Verification items for this drawing (mm, ordinates from the low corner). Give positions to 0.01 mm unless a question says otherwise; leave off trailing zeros. Loops run counter-clockwise (first coordinate to the right, second up) from the corner with the lowest first, then second, coordinate; pieces in that order, holes last. Notation, with made-up numbers: M -6,-16.5 L 0,-16.5 A30 ccw 0,20.5 Z; hole C 10.25,35 d10. An arc over 180 degrees is marked long. Use a Markdown table: item, result.
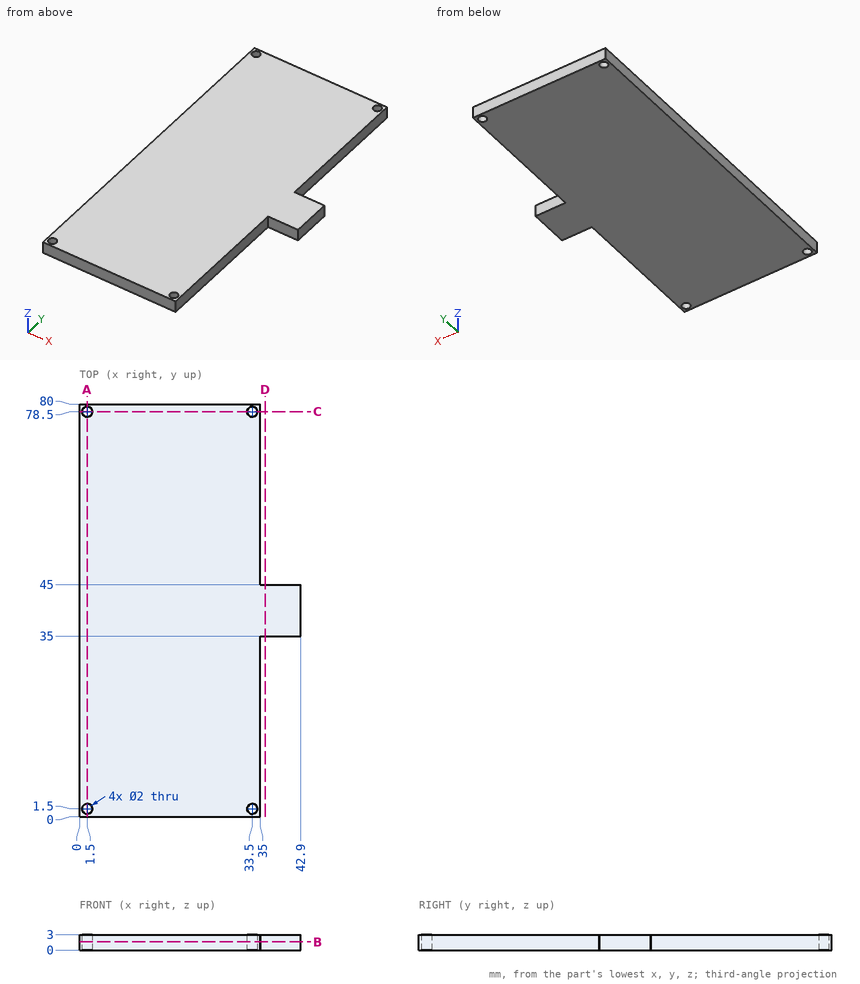
(1) Gauge pin test, flat end, axial feed: P1, Ø1.8, axis at x = 33.5, y = 1.5, coming from the +Z side. Record the tip position at first contact, or that the pin passes through.
Results below:
| item | result |
|---|---|
| P1 | through |
(2) Material ranges on line 1 (Y direction, x = 33.5, z = 1.45); line 2 (X direction, y = 78.5, z = 1.35); line 3 (X direction, y = 32, z = 0.5), recorded low to high.
Results below:
| item | result |
|---|---|
| line 1 | 0 to 0.5, 2.5 to 77.5, 79.5 to 80 |
| line 2 | 0 to 0.5, 2.5 to 32.5, 34.5 to 35 |
| line 3 | 0 to 35 |
(3) Cross-section at B-B on z = 1.6. Record the cut outline in (x, y).
Results below:
| item | result |
|---|---|
| outline | M 0,0 L 35,0 L 35,35 L 42.9,35 L 42.9,45 L 35,45 L 35,80 L 0,80 Z; hole C 1.5,1.5 d2; hole C 1.5,78.5 d2; hole C 33.5,1.5 d2; hole C 33.5,78.5 d2 |
(4) Cross-section at C-C on y = 78.5. Record the cut outline in (x, z).
Results below:
| item | result |
|---|---|
| outline | M 0,0 L 0.5,0 L 0.5,3 L 0,3 Z; M 2.5,0 L 32.5,0 L 32.5,3 L 2.5,3 Z; M 34.5,0 L 35,0 L 35,3 L 34.5,3 Z |
(5) Cross-section at A-A on x = 1.5. Record the cut outline in (y, z), then the cut area to 3 significant figures.
Results below:
| item | result |
|---|---|
| outline | M 0,0 L 0.5,0 L 0.5,3 L 0,3 Z; M 2.5,0 L 77.5,0 L 77.5,3 L 2.5,3 Z; M 79.5,0 L 80,0 L 80,3 L 79.5,3 Z |
| area | 228 mm^2 |
(6) Cross-section at D-D on x = 36. Record the cut outline in (y, z).
Results below:
| item | result |
|---|---|
| outline | M 35,0 L 45,0 L 45,3 L 35,3 Z |
